```python
from build123d import *

# Parameters (mm, degrees)
SKETCH1_W           = 76.2
SKETCH1_H           = 19.05
SKETCH1_R           = 2.38
BOSS_EXTRUDE1_DEPTH = 6.35


with BuildPart() as part:
    # Sketch1 → Boss-Extrude1 (new body)
    with BuildSketch(Plane(origin=(0, 0, 0), x_dir=(1, 0, 0), z_dir=(0, 1, 0))):
        with Locations((0, 9.525)):
            Rectangle(SKETCH1_W, SKETCH1_H)
        with Locations((-28.75, 9.525)):
            Circle(SKETCH1_R, mode=Mode.SUBTRACT)
        with BuildLine():
            Line((33.34, 13.514849621), (33.34, 5.535150379))
            ThreePointArc((33.34, 5.535150379), (22.05, 9.525), (33.34, 13.514849621))
        make_face(mode=Mode.SUBTRACT)
    extrude(amount=BOSS_EXTRUDE1_DEPTH)


solid = part.part
```
Build history of the part. All positions in model axes, mm. A direction names the side the tool comes from. Coordinates: 2 decimals unless noted, no trailing zeros. Order: outer loops, then holes, each group sorted by start corner. A loop starts at its lowest first (then second) coordinate and runs counter-clockwise, first axis right, second up. Notation, with made-up numbers: (10, -5) -> (36, -5) arc R20 ccw to (36, 24) -> close; hole circle Ø6 at (-6.75, 4). An arc over 180 degrees is marked (long way). Answer in a Markdown table with one row per item. Add a question column.
Q1. Mould opens along Z. For faces 1 (the face through (22.054, 3.131, -9.306)), 2 (the face through (-1, 3, 0)), 3 (the face through (-1, 3, -19.05)), 4 (the face through (38.1, 3, -9)) say: +Z half, -Z half, draft (parallel to the pull), parting line (faces both ways), or undercut.
Q2. Band-saw the part on C-C, the plane z = -15. List the corners of the cut face in (x, y).
Q3. Band-saw the part on A-A, the plane x = 28.4. List the corners of the cut face in (y, z) (3 decimals), then the cut area to 3 significant figures.
Q4. Wall check: line 1 along Z through (x, y) = (28.4, 4.75) (3 decimals); line 2 along X through (y, z) = (4, -11.25); line 3 along X through (y, z) = (6, -7.5). Give the ranges that are in metal, low to high. Write a range as [from, to].
Q5. Band-saw the part on B-B, the plane y = 3.5. List the corners of the cut face in (x, z) (3 decimals).
Q6. Which spindle directions (+Z, -Z, +X, -X, +Y, -Y) get a long thin tool onto all of the face, cutting with end or side? Do faces 5 (the face through (-1, 0, -10)), 6 (the face through (33.34, 3, -10)). Say none if no direction does.
Answers follow:
| question | item | result |
|---|---|---|
| 1 | face 1 | undercut |
| 1 | face 2 | +Z half |
| 1 | face 3 | -Z half |
| 1 | face 4 | draft |
| 2 | outline | (-38.1, 0) -> (25.18, 0) -> (25.18, 6.35) -> (-38.1, 6.35) -> close; (31.62, 0) -> (38.1, 0) -> (38.1, 6.35) -> (31.62, 6.35) -> close |
| 3 | outline | (0, -19.05) -> (6.35, -19.05) -> (6.35, -15.875) -> (0, -15.875) -> close; (0, -3.175) -> (6.35, -3.175) -> (6.35, 0) -> (0, 0) -> close |
| 3 | area | 40.3 mm^2 |
| 4 | line 1 | [-19.05, -15.875], [-3.175, 0] |
| 4 | line 2 | [-38.1, -30.39], [-27.11, 22.29], [33.34, 38.1] |
| 4 | line 3 | [-38.1, -30], [-27.5, 22.38], [33.34, 38.1] |
| 5 | outline | (-38.1, -19.05) -> (38.1, -19.05) -> (38.1, 0) -> (-38.1, 0) -> close; hole circle Ø4.76 at (-28.75, -9.525); hole (33.34, -13.515) -> (33.34, -5.535) arc R6.35 ccw (long way) to start |
| 6 | face 5 | +Z, -Z, +X, -X, -Y |
| 6 | face 6 | +Y, -Y |
